The model under review builds one solid part; all positions refer to its coordinate system, in mm. Coordinates: 2 decimals unless noted, no trailing zeros. Write each loop counter-clockwise with the first axis right and the second up, starting at its lowest first coordinate (ties: lowest second). Pieces come first, ordered by that corner, then holes.
1) For line 1 (Z direction, x = 0.7, y = 1.55); line 2 (Y direction, x = -1.35, z = -1.5); line 3 (X direction, y = -0.15, z = 8), list the stretches that pass through material, from the lowest coordinate up.
2) Add section A-A, the plane x = 0. State the section outline as (y, z) points, then the cut area to 3 significant figures.
3) Add section C-C, the plane z = -19.5. State the section outline as (x, y) points.
from build123d import *

# Parameters (mm, degrees)
SKETCH1_R           = 1.8542
BOSS_EXTRUDE1_DEPTH = 25.4
SKETCH2_R           = 1.2827
BOSS_EXTRUDE2_DEPTH = 7.62
SKETCH3_R           = 1.2827
CUT_EXTRUDE1_DEPTH  = 2.54


with BuildPart() as part:
    # Sketch1 → Boss-Extrude1 (new, symmetric)
    with BuildSketch(Plane.XY):
        Circle(SKETCH1_R)
    extrude(amount=BOSS_EXTRUDE1_DEPTH, both=True)

    # Sketch2 → Boss-Extrude2 (add)
    with BuildSketch(Plane.XY.offset(25.4)):
        with Locations(Location((0, 0, 0), (0, 0, 180))):
            Circle(SKETCH2_R)
    boss_extrude2 = extrude(amount=BOSS_EXTRUDE2_DEPTH)

    # Mirror1: Boss-Extrude2 across plane
    add(boss_extrude2.mirror(Plane.XY))

    # Sketch3 → Cut-Extrude1 (cut)
    with BuildSketch(Plane.XY.offset(33.02)):
        with Locations(Location((0, 0, 0), (0, 0, 180))):
            Circle(SKETCH3_R)
    extrude(amount=-CUT_EXTRUDE1_DEPTH, mode=Mode.SUBTRACT)


solid = part.part
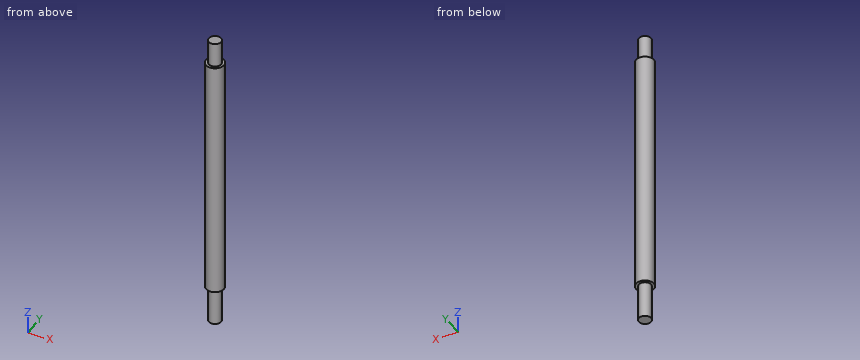
Geometry results:
1. line 1: z = -25.4 to 25.4
1. line 2: y = -1.27 to 1.27
1. line 3: x = -1.85 to 1.85
2. outline: (-1.85, -25.4) - (-1.28, -25.4) - (-1.28, -33.02) - (1.28, -33.02) - (1.28, -25.4) - (1.85, -25.4) - (1.85, 25.4) - (1.28, 25.4) - (1.28, 30.48) - (-1.28, 30.48) - (-1.28, 25.4) - (-1.85, 25.4) - close
2. area: 221 mm2
3. outline: circle Ø3.71 at (0, 0)
